Autodesk Inventor part; units mm, degrees
ref_plane "YZ Plane" through (0, 0, 0) normal (1, 0, 0) x (0, 1, 0)
ref_plane "XZ Plane" through (0, 0, 0) normal (0, 1, 0) x (-1, 0, 0)
ref_plane "XY Plane" through (0, 0, 0) normal (0, 0, 1) x (1, 0, 0)
sketch "Sketch1" plane through (0, 0, 0) normal (0, 0, 1) x (1, 0, 0)
  circle A0 centre (-50.6259, -62.1376) radius 2.067
  circle A1 centre (-60.6259, -62.1376) radius 2.067
  circle A2 centre (-70.6259, -62.1376) radius 2.067
  arc A3 (-51.6259, -32.7366) -> (-51.6259, -28.7366) centre (-51.6259, -30.7366) ccw
  line L0 (-51.6259, -32.7366) -> (-61.6259, -32.7366)
  arc A4 (-61.6259, -28.7366) -> (-61.6259, -32.7366) centre (-61.6259, -30.7366) ccw
  line L1 (-61.6259, -28.7366) -> (-51.6259, -28.7366)
  circle A5 centre (-47.1259, -20.7366) radius 1.2295
  circle A6 centre (-66.1259, -20.7366) radius 1.2295
  circle A7 centre (-47.1259, -10.7366) radius 1.2295
  circle A8 centre (-66.1259, -10.7366) radius 1.2295
  circle A9 centre (-33.2634, 4.8443) radius 1.2295
  circle A10 centre (-15.9429, 14.8443) radius 1.2295
  circle A11 centre (1.3776, 24.8443) radius 1.2295
  circle A12 centre (18.6981, 34.8443) radius 1.2295
  circle A13 centre (36.0187, 44.8443) radius 1.2295
  circle A14 centre (53.3392, 54.8443) radius 1.2295
  circle A15 centre (70.6597, 64.8443) radius 1.2295
  line L2 (72.8006, 71.2078) -> (72.645, 71.1179)
  arc A16 (72.645, 71.1179) -> (69.1955, 71.4356) centre (70.6956, 68.8376) ccw
  line L3 (69.1955, 71.4356) -> (-42.6259, 6.8679)
  line L4 (-42.6259, 6.8679) -> (-42.6259, 0.2634)
  arc A17 (-48.6259, -5.7366) -> (-42.6259, 0.2634) centre (-48.6259, 0.2634) ccw
  line L5 (-48.6259, -5.7366) -> (-67.6259, -5.7366)
  arc A18 (-67.6259, -5.7366) -> (-72.6259, -10.7366) centre (-67.6259, -10.7366) ccw
  line L6 (-72.6259, -10.7366) -> (-72.6259, -46.4376)
  arc A19 (-78.6259, -52.4376) -> (-72.6259, -46.4376) centre (-78.6259, -46.4376) ccw
  line L7 (-78.6259, -52.4376) -> (-78.6259, -71.8376)
  line L8 (-78.6259, -71.8376) -> (-48.6259, -71.8376)
  arc A20 (-48.6259, -71.8376) -> (-23.6259, -46.8376) centre (-48.6259, -46.8376) ccw
  arc A21 (16.3839, 22.4655) -> (-23.6259, -46.8376) centre (56.4008, -46.8376) ccw
  line L9 (16.3839, 22.4655) -> (77.126, 57.5391)
  arc A22 (77.126, 57.5391) -> (78.2359, 61.6161) centre (75.6259, 60.1371) ccw
  line L10 (78.2359, 61.6161) -> (72.8006, 71.2078)
  line L11 (-78.6259, -52.4376) -> (-46.6259, -52.4376)
  line L12 (-46.6259, -52.4376) -> (-46.6259, -71.8376)
  line L13 (-46.6259, -71.8376) -> (-78.6259, -71.8376)
  line L14 (-78.6259, -71.8376) -> (-78.6259, -52.4376)
  circle A23 centre (-70.6259, -62.1376) radius 2.6
  circle A24 centre (-60.6259, -62.1376) radius 2.6
  circle A25 centre (-50.6259, -62.1376) radius 2.6
  point P0 (0, 0)
  point P1 (-46.6259, -71.7575)
  dimension "d0" = 32
  dimension "d1" = 19.4
  dimension "d2" = 5.2
  dimension "d3" = 5.2
  dimension "d4" = 5.2
extrude "Extrusion1" add sketch "Sketch1" along normal blind 29 contours L12 L13 A20 | A20 L8 L7 L11 L12
sketch "Sketch2" plane through (-46.6259, -71.7575, 0) normal (1, 0, 0) x (0, 0, -1)
  circle A0 centre (-21.95, 17.1199) radius 1.25
  circle A1 centre (-21.95, 2.1199) radius 1.25
  circle A2 centre (-5.95, 2.1199) radius 1.25
  circle A3 centre (-5.95, 17.1199) radius 1.25
  point P0 (0, 71.7575)
hole "Hole1" at (-46.6259, -69.6376, 21.95) at (-46.6259, -69.6376, 5.95) at (-46.6259, -54.6376, 5.95) at (-46.6259, -54.6376, 21.95) direction (-1, 0, 0) diameter 3.4 end through all
properties part number "connection block mgn9h"
Geometry: final body of the model. Coordinates: model frame, mm. Give positions to 0.01 mm unless a question says otherwise; leave off trailing zeros. Write each loop counter-clockwise with the first axis right and the second up, starting at its lowest first coordinate (ties: lowest second). Pieces come first, ordered by that corner, then holes.
1. Section query D-D, the plane y = -61. Return loops of the section in (x, z).
2. Pin query (flat end, axial travel): P1, Ø3, axis at x = -70.63, y = -62.14, coming from the +Z side. Return the tip coordinate at first contact, or that it passes through.
3. Section query B-B, the plane x = -58.5. Return loops of the section in (y, z).
4. Draft query along Y for faces 1 (the flat face through (-62, -71.838, 14)), 2 (the flat face through (-63, -52.438, 14)), 3 (the cylindrical face through (-62.85, -53.603, 23.299)). Return one class per face: released by +Y, released by -Y, zero draft, split by the parting line, or undercut.
5. Section query A-A, the plane z = 21.25. Return loops of the section in (x, y).
6. Line query: probe 1 along Y at (x, z) = (-54, 5.95); probe 2 along Y at (x, z) = (-72, 23.25); probe 3 along X at (y, z) = (-63.75, 22.5). Output: solid intervals per line, ascending.
7. Section query C-C, the plane x = -67. Return loops of the section in (y, z), then the cut area to 3 significant figures.
Computed:
1. outline: (-78.63, 0) - (-72.96, 0) - (-72.96, 29) - (-78.63, 29) - close; (-68.29, 0) - (-62.96, 0) - (-62.96, 29) - (-68.29, 29) - close; (-58.29, 0) - (-52.96, 0) - (-52.96, 29) - (-58.29, 29) - close; (-48.29, 0) - (-46.63, 0) - (-46.63, 29) - (-48.29, 29) - close
2. P1: passes through
3. outline: (-71.84, 0) - (-63.63, 0) - (-63.63, 29) - (-71.84, 29) - close; (-60.64, 0) - (-52.44, 0) - (-52.44, 29) - (-60.64, 29) - close; hole circle Ø3.4 at (-69.64, 5.95); hole circle Ø3.4 at (-69.64, 21.95); hole circle Ø3.4 at (-54.64, 5.95); hole circle Ø3.4 at (-54.64, 21.95)
4. face 1: released by -Y
4. face 2: released by +Y
4. face 3: undercut
5. outline: (-78.63, -71.84) - (-46.63, -71.84) - (-46.63, -71.19) - (-78.63, -71.19) - close; (-78.63, -68.09) - (-46.63, -68.09) - (-46.63, -56.19) - (-78.63, -56.19) - close; (-78.63, -53.09) - (-46.63, -53.09) - (-46.63, -52.44) - (-78.63, -52.44) - close; hole circle Ø5.2 at (-70.63, -62.14); hole circle Ø5.2 at (-60.63, -62.14); hole circle Ø5.2 at (-50.63, -62.14)
6. probe 1: y = -71.84 to -71.34, -67.94 to -56.34, -52.94 to -52.44
6. probe 2: y = -71.84 to -70.73, -68.54 to -64.34, -59.93 to -55.73, -53.54 to -52.44
6. probe 3: x = -78.63 to -72.67, -68.59 to -62.67, -58.59 to -52.67, -48.59 to -46.63
7. outline: (-71.84, 0) - (-52.44, 0) - (-52.44, 29) - (-71.84, 29) - close; hole circle Ø3.4 at (-69.64, 5.95); hole circle Ø3.4 at (-69.64, 21.95); hole circle Ø3.4 at (-54.64, 5.95); hole circle Ø3.4 at (-54.64, 21.95)
7. area: 526 mm2
